Can you work these out from the drawing? Everything is in mm from the part's minimum corner. A direction names the side the tool comes from. Round coordinates to 2 decimals unless told otherwise and drop trailing zeros. Loops run counter-clockwise (first coordinate to the right, second up) from the corner with the lowest first, then second, coordinate; pieces in that order, holes last. Notation, with made-up numbers: (-1.5, 31) - (41.5, 31) arc R9 cw to (41.5, 48) - close; hole circle Ø10 at (-2.5, 39.25). An arc over 180 degrees is marked (long way). Answer as CSV lines item,"result". Start each with the question number.
1) I'm going to push flat-ended pins straight in: pin 1 Ø4 at (x, z) = (14.5, 6.5) entering from -Y; pin 2 Ø2.5 at (x, y) = (13, 5) entering from +Z; pin 3 Ø1.8 at (x, z) = (18.5, 13.2) entering from +Y. Where does each tip first touch, or does it pass through?
2) Suppose I cut it at A-A, the plane z = 13.2. Write out the boundary of the cut face in (x, y), then the cut area to 3 significant figures.
3) Which directions (+Z, -Z, +X, -X, +Y, -Y) give clear straight access to the entire face, cutting with the end or side of a thin tool? Please do the marked faces 1 and 2.
4) Please list where these lines run through material, in increasing order: line 1 along X through (y, z) = (8.4, 13.2); line 2 along Z through (x, y) = (2.5, 2.5); line 3 along Y through (x, z) = (13.75, 2.75).
5) Suppose I cut it at C-C, the plane y = 5. Write out the boundary of the cut face in (x, z), then the cut area to 3 significant figures.
6) Suppose I cut it at D-D, the plane x = 16. Write out the boundary of the cut face in (y, z), then the cut area to 4 significant figures.
7) Suppose I cut it at B-B, the plane x = 18.5. Write out the boundary of the cut face in (y, z), then the cut area to 4 significant figures.
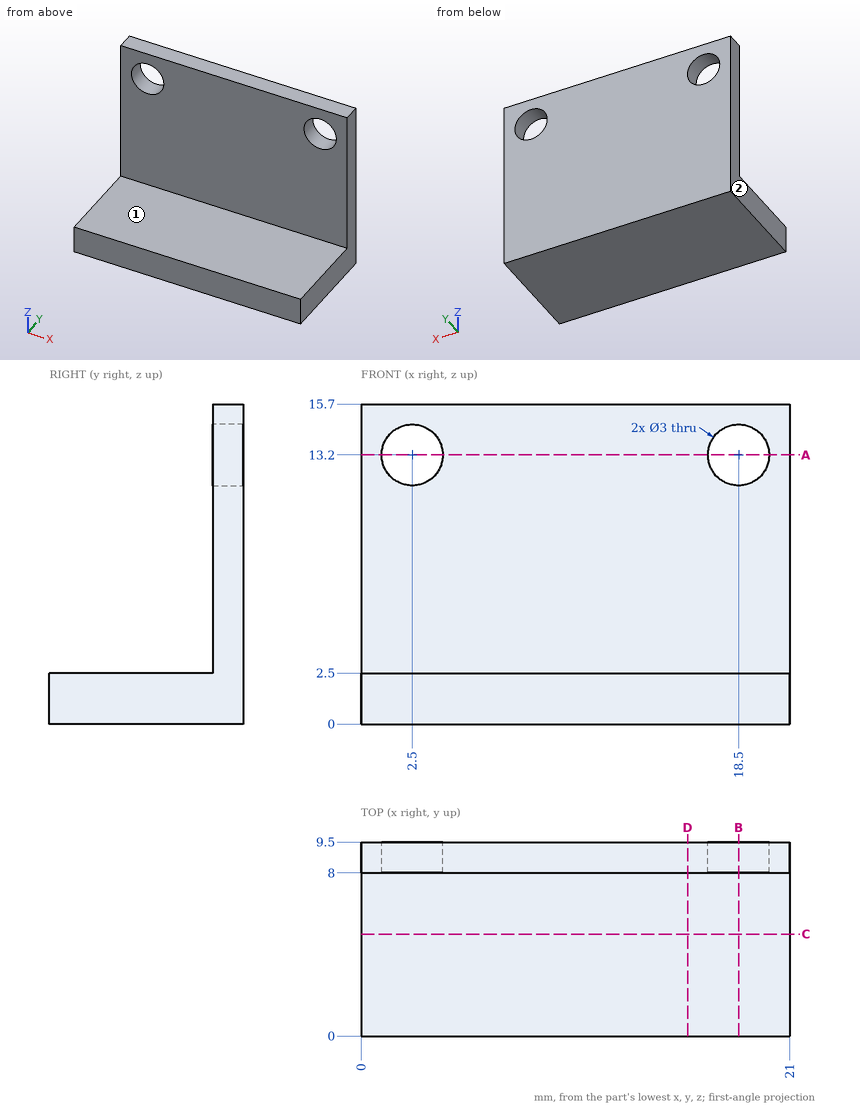
Filled sheet:
1,pin 1,"y = 8"
1,pin 2,"z = 2.5"
1,pin 3,"through"
2,outline,"(0, 8) - (1, 8) - (1, 9.5) - (0, 9.5) - close; (4, 8) - (17, 8) - (17, 9.5) - (4, 9.5) - close; (20, 8) - (21, 8) - (21, 9.5) - (20, 9.5) - close"
2,area,"22.5 mm²"
3,face 1,"+Z, +X, -X, -Y"
3,face 2,"+Z, -Z, -X, +Y, -Y"
4,line 1,"0 to 1, 4 to 17, 20 to 21"
4,line 2,"0 to 2.5"
4,line 3,"8 to 9.5"
5,outline,"(0, 0) - (21, 0) - (21, 2.5) - (0, 2.5) - close"
5,area,"52.5 mm²"
6,outline,"(0, 0) - (9.5, 0) - (9.5, 15.7) - (8, 15.7) - (8, 2.5) - (0, 2.5) - close"
6,area,"43.55 mm²"
7,outline,"(0, 0) - (9.5, 0) - (9.5, 11.7) - (8, 11.7) - (8, 2.5) - (0, 2.5) - close; (8, 14.7) - (9.5, 14.7) - (9.5, 15.7) - (8, 15.7) - close"
7,area,"39.05 mm²"
